Design review of the part built by this model. Coordinates are the model's own, in mm. Face numbers are marked on the shaded views. A direction names the side the tool comes from. Give positions to 0.01 mm unless a question says otherwise; leave off trailing zeros. Loops run counter-clockwise (first coordinate to the right, second up) from the corner with the lowest first, then second, coordinate; pieces in that order, holes last. Notation, with made-up numbers: (14, 72) - (61, 72) arc R19 cw to (61, 94) - close; hole circle Ø2 at (-0.75, -31.75). An arc over 180 degrees is marked (long way). Write each question's results on one line, items separated by ' | '.
```python
from build123d import *

# Parameters (mm, degrees)
SKIZZE2_R                       = 1
SCHNITT_LINEAR_AUSTRAGEN1_DEPTH = 10
SKIZZE2_3_R                     = 1.25
SKIZZE2_3_R_2                   = 1
SCHNITT_LINEAR_AUSTRAGEN2_DEPTH = 2
SKIZZE3_R                       = 1.25
SCHNITT_LINEAR_AUSTRAGEN3_DEPTH = 4.05


with BuildPart() as part:
    # Skizze1 → Rotation1 (revolve)
    with BuildSketch(Plane.XY):
        Polygon((-11, 3), (-8, 3), (-8, 3.05), (8, 3.05), (8, 3), (11, 3), (11, 0), (-11, 0), align=None)
    revolve(axis=Axis((-97.111770595, 0, 0), (-1, 0, 0)))

    # Skizze2 → Schnitt-Linear austragen1 (cut)
    with BuildSketch(Plane(origin=(11, 0, 0), x_dir=(0, 0, -1), z_dir=(1, 0, 0))):
        Circle(SKIZZE2_R)
    extrude(amount=-SCHNITT_LINEAR_AUSTRAGEN1_DEPTH, mode=Mode.SUBTRACT)

    # Skizze2<3> → Schnitt-Linear austragen2 (cut)
    with BuildSketch(Plane(origin=(11, 0, 0), x_dir=(0, 0, -1), z_dir=(1, 0, 0))):
        Circle(SKIZZE2_3_R)
        Circle(SKIZZE2_3_R_2, mode=Mode.SUBTRACT)
    extrude(amount=-SCHNITT_LINEAR_AUSTRAGEN2_DEPTH, mode=Mode.SUBTRACT)

    # Skizze3 → Schnitt-Linear austragen3 (cut, through all)
    with BuildSketch(Plane(origin=(0, 0, 0), x_dir=(1, 0, 0), z_dir=(0, 1, 0))):
        with Locations((4.5, 0)):
            Circle(SKIZZE3_R)
    extrude(amount=SCHNITT_LINEAR_AUSTRAGEN3_DEPTH, mode=Mode.SUBTRACT)


solid = part.part
```
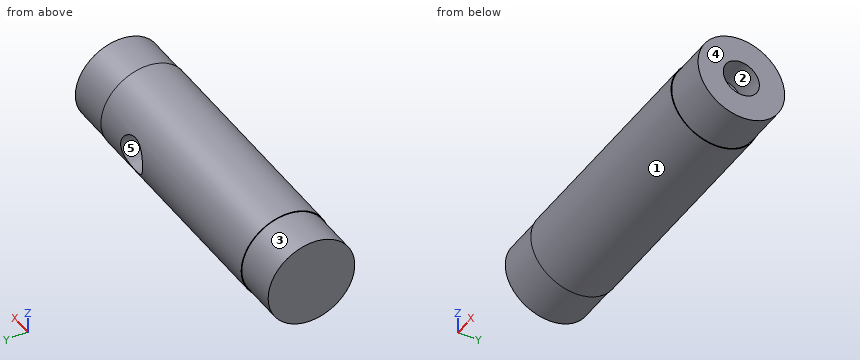
Item 1: Tool access review of the marked faces 1 and 2: name each direction out of +Z, -Z, +X, -X, +Y, -Y from which nothing blocks a thin tool from reaching the whole face with its end or side.
Output values:
face 1: +X, -X | face 2: +X
Item 2: We need section C-C on z = 1.5. Give the boundary of the cut face in (x, y), then the cut area to 3 significant figures.
Output values:
outline: (-11, -2.6) - (-8, -2.6) - (-8, -2.66) - (8, -2.66) - (8, -2.6) - (11, -2.6) - (11, 2.6) - (8, 2.6) - (8, 2.66) - (-8, 2.66) - (-8, 2.6) - (-11, 2.6) - close | area: 116 mm²
Item 3: We need section D-D on y = 0.25. Give the boundary of the cut face in (x, z), then the cut area to 3 significant figures.
Output values:
outline: (-11, -2.99) - (-8, -2.99) - (-8, -3.04) - (8, -3.04) - (8, -2.99) - (11, -2.99) - (11, -1.22) - (9, -1.22) - (9, -0.97) - (5.29, -0.97) arc R1.25 cw to (3.71, -0.97) - (1, -0.97) - (1, 0.97) - (3.71, 0.97) arc R1.25 cw to (5.29, 0.97) - (9, 0.97) - (9, 1.22) - (11, 1.22) - (11, 2.99) - (8, 2.99) - (8, 3.04) - (-8, 3.04) - (-8, 2.99) - (-11, 2.99) - close | area: 112 mm²
Item 4: We need section A-A on z = 0. Give the boundary of the cut face in (x, y).
Output values:
outline: (-11, -3) - (-8, -3) - (-8, -3.05) - (8, -3.05) - (8, -3) - (11, -3) - (11, -1.25) - (9, -1.25) - (9, -1) - (1, -1) - (1, 1) - (3.25, 1) - (3.25, 3.05) - (-8, 3.05) - (-8, 3) - (-11, 3) - close; (5.75, 1) - (9, 1) - (9, 1.25) - (11, 1.25) - (11, 3) - (8, 3) - (8, 3.05) - (5.75, 3.05) - close
Item 5: We need section B-B on y = 1.5. Give the boundary of the cut face in (x, z), then the cut area to 3 significant figures.
Output values:
outline: (-11, -2.6) - (-8, -2.6) - (-8, -2.66) - (8, -2.66) - (8, -2.6) - (11, -2.6) - (11, 2.6) - (8, 2.6) - (8, 2.66) - (-8, 2.66) - (-8, 2.6) - (-11, 2.6) - close; hole circle Ø2.5 at (4.5, 0) | area: 111 mm²
Item 6: Wall thickness on probe 1 along X at (y, z) = (1.2, 0); probe 2 along X at (y, z) = (1, -1); probe 3 along Y at (x, z) = (9.55, 0): over which ranges is each line inside the solid? List them lowest first.
Output values:
probe 1: x = -11 to 3.25, 5.75 to 9 | probe 2: x = -11 to 3.75, 5.25 to 11 | probe 3: y = -3 to -1.25, 1.25 to 3
Item 7: Draft analysis for pull direction Z (two halves, no side actions). For the marked faces 3, 4 and 5, state which applies: +Z half, -Z half, draft (parallel to the pull), parting line (faces both ways), or undercut.
Output values:
face 3: parting line | face 4: draft | face 5: undercut
